from build123d import *

# Parameters (mm, degrees)
SKETCH_1_W      = 8
SKETCH_1_H      = 8
SKETCH_1_R      = 2
EXTRUDE_1_DEPTH = 4
FILLET_1_R      = 1


with BuildPart() as part:
    # 草图1 → 凸台-拉伸1 (new body)
    with BuildSketch(Plane(origin=(0, 0, 0), x_dir=(1, 0, 0), z_dir=(0, 1, 0))):
        Rectangle(SKETCH_1_W, SKETCH_1_H)
        Circle(SKETCH_1_R, mode=Mode.SUBTRACT)
    extrude(amount=EXTRUDE_1_DEPTH)

    # 圆角1
    fillet_1_edges = [part.edges().sort_by_distance(p)[0] for p in [
        (4, 2, 4),
        (-4, 2, 4),
        (-4, 2, -4),
        (4, 2, -4),
    ]]
    fillet(fillet_1_edges, radius=FILLET_1_R)


solid = part.part
Source: CAD feature listing. Evaluate the final solid. Frame: model axes, mm. Give positions to 0.01 mm unless a question says otherwise; leave off trailing zeros. Loops run counter-clockwise (first coordinate to the right, second up) from the corner with the lowest first, then second, coordinate; pieces in that order, holes last. Notation, with made-up numbers: (14.25, -37) -> (57.25, -37) arc R20 cw to (57.25, -3) -> close; hole circle Ø3 at (32, -26). An arc over 180 degrees is marked (long way). Use a Markdown table: item, result. Add a question column.
1) Line query: line 1 along Z through (x, y) = (0, 2); line 2 along Z through (x, y) = (1.5, 3.8). Output: solid intervals per line, ascending. Write a range as [from, to].
2) Section query D-D, the plane x = 3.5. Return the cut outline in (y, z).
3) Section query B-B, the plane z = 0. Return the cut outline in (x, y).
4) Section query C-C, the plane y = 0.35. Return the cut outline in (x, z).
5) Pull-direction query (Z, two-part tool) for faces 1 (the face through (-2, 4, -1)), 2 (the face through (-3.715, 2.028, 3.699)), 3 (the face through (0, 2, 2)), 4 (the face through (3.699, 2.028, -3.715)); classes: +Z half, -Z half, draft (parallel to the pull), parting line (faces both ways), or undercut.
6) Section query A-A, the plane x = 0. Return the cut outline in (y, z), then the cut area to 3 significant figures.
Numbers:
| question | item | result |
|---|---|---|
| 1 | line 1 | z = [-4, -2], [2, 4] |
| 1 | line 2 | z = [-4, -1.32], [1.32, 4] |
| 2 | outline | (0, -3.87) -> (4, -3.87) -> (4, 3.87) -> (0, 3.87) -> close |
| 3 | outline | (-4, 0) -> (-2, 0) -> (-2, 4) -> (-4, 4) -> close; (2, 0) -> (4, 0) -> (4, 4) -> (2, 4) -> close |
| 4 | outline | (-4, -3) arc R1 ccw to (-3, -4) -> (3, -4) arc R1 ccw to (4, -3) -> (4, 3) arc R1 ccw to (3, 4) -> (-3, 4) arc R1 ccw to (-4, 3) -> close; hole circle Ø4 at (0, 0) |
| 5 | face 1 | draft |
| 5 | face 2 | +Z half |
| 5 | face 3 | undercut |
| 5 | face 4 | -Z half |
| 6 | outline | (0, -4) -> (4, -4) -> (4, -2) -> (0, -2) -> close; (0, 2) -> (4, 2) -> (4, 4) -> (0, 4) -> close |
| 6 | area | 16.0 mm2 |
